For this review, take the finished solid that the model builds, in its own axes (mm). Face numbers are marked on the shaded views. A direction names the side the tool comes from. Round coordinates to 2 decimals unless told otherwise and drop trailing zeros. Loops run counter-clockwise (first coordinate to the right, second up) from the corner with the lowest first, then second, coordinate; pieces in that order, holes last.
1. Draft analysis for pull direction X (two halves, no side actions). For the marked faces 3, 4 and 5, state which applies: released by +X, released by -X, zero draft, split by the parting line, or undercut.
2. To check wall thickness, follow line 1 along Y through (x, z) = (71, 22); line 2 along X through (y, z) = (13, 22) (3 decimals); line 3 along X through (y, z) = (43, 4.75). State the ranges of each line that lie inside material, in increasing order.
3. Tool access review of the marked faces 1 and 2: name each direction out of +Z, -Z, +X, -X, +Y, -Y from which nothing blocks a thin tool from reaching the whole face with its end or side.
4. Consider section B-B on x = 75. State the section outline as (y, z) points.
5. Clearance check with flat-ended pins moving along their axes: pin 1 Ø2 at (x, z) = (45, 24) entering from +Y; pin 2 Ø4 at (x, z) = (18, 22) entering from +Y; pin 3 Ø1.5 at (x, z) = (55.5, 10) entering from -Y; pin 4 Ø8 at (x, y) = (18, 10) entering from +Z. State where each tip first meets the part, or that it passes through.
6. Consider section A-A on z = 19. State the section outline as (x, y) points (3 decimals), then the cut area to 3 significant figures.
7. Consider section C-C on y = 18.5. State the section outline as (x, z) points (3 decimals).
Solid Edge part; units mm, degrees
sketch "Sketch1" plane through (0, 0, 0) normal (0, 0, 1) x (1, 0, 0)
  line L0 (-0.015, 0.026) -> (1.985, 0.026)
  line L1 (1.985, 0.026) -> (1.985, 15.026)
  arc A0 (1.985, 15.026) -> (67.485, 80.526) centre (1.985, 80.526) ccw
  line L2 (82.485, 80.526) -> (67.485, 80.526)
  line L3 (82.485, 82.526) -> (82.485, 80.526)
  line L4 (62.485, 82.526) -> (82.485, 82.526)
  arc A1 (62.485, 82.526) -> (-0.015, 20.026) centre (-0.015, 82.526) cw
  line L5 (-0.015, 0.026) -> (-0.015, 20.026)
extrude "Protrusion1" add sketch "Sketch1" along normal blind 30
extrude "ExtrudedCutout_1" [suppressed]
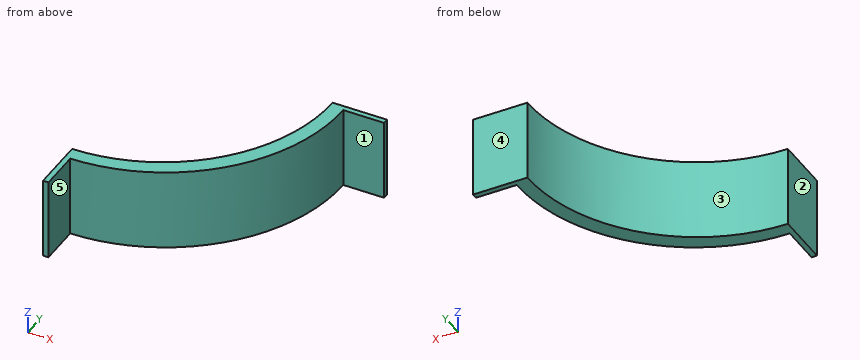
Resolved:
1. face 3: released by -X
1. face 4: zero draft
1. face 5: released by +X
2. line 1: y = 80.53 to 82.53
2. line 2: x = -0.015 to 1.985
2. line 3: x = 48.4 to 55.67
3. face 1: +Z, -Z, +X, -Y
3. face 2: +Z, -Z, -X, +Y, -Y
4. outline: (80.53, 0) - (82.53, 0) - (82.53, 30) - (80.53, 30) - close
5. pin 1: stops at y = 40.23
5. pin 2: stops at y = 23.32
5. pin 3: stops at y = 41.72
5. pin 4: passes through
6. outline: (-0.015, 0.026) - (1.985, 0.026) - (1.985, 15.026) arc R65.5 ccw to (67.485, 80.526) - (82.485, 80.526) - (82.485, 82.526) - (62.485, 82.526) arc R62.5 cw to (-0.015, 20.026) - close
6. area: 628 mm2
7. outline: (-0.015, 0) - (23.033, 0) - (23.033, 30) - (-0.015, 30) - close
